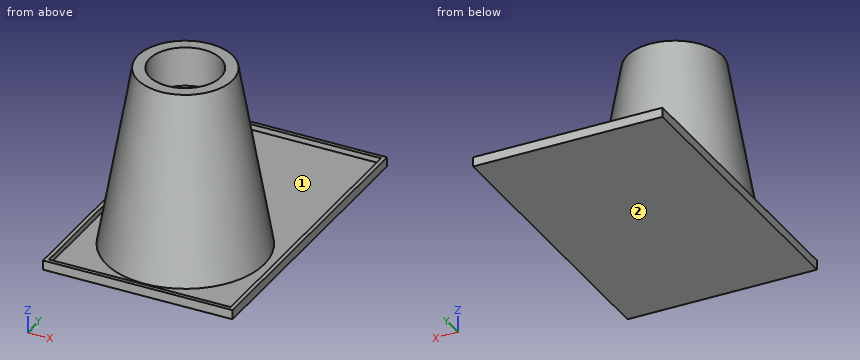
from build123d import *

# Parameters (mm, degrees)
F0_W     = 120
F0_H     = 190
F1_DEPTH = 6
F2_T     = -2.5
F3_R     = 50
F4_DEPTH = 115
F5_SIZE2 = 114.99999
F5_SIZE  = 19.99999
F6_R     = 22.5
F7_DEPTH = 25


# Not quite as in the source:
# - a fillet or chamfer is up to 0.001 mm smaller than in the source, because OpenCascade refuses the exact size


with BuildPart() as f1:
    # F0 (on Top) → F1 (new body)
    with BuildSketch(Plane.XY):
        with Locations((0, 36.5384568274)):
            Rectangle(F0_W, F0_H)
    extrude(amount=F1_DEPTH)

    # F2
    f2_openings = [f1.faces().sort_by_distance(p)[0] for p in [
        (0, 36.538457, 6),
    ]]
    offset(amount=F2_T, openings=f2_openings)

    # F3 (on face) → F4 (join)
    with BuildSketch(Plane.XY.offset(2.5)):
        Circle(F3_R)
    extrude(amount=F4_DEPTH)

    # F5 (size 20 and 115 in the source; OpenCascade refuses exactly that, so slightly less here)
    f5_edges = [f1.edges().sort_by_distance(p)[0] for p in [
        (-50, 0, 117.5),
    ]]
    f5_side = f1.faces().sort_by_distance((0, 0, 117.5))[0]
    chamfer(f5_edges, length=F5_SIZE, length2=F5_SIZE2, reference=f5_side)

    # F6 (on face) → F7 (cut)
    with BuildSketch(Plane.XY.offset(117.5)):
        Circle(F6_R)
    extrude(amount=-F7_DEPTH, mode=Mode.SUBTRACT)


solid = f1.part
The listing builds one solid part. Answer for the finished solid, in the listing's coordinates (mm). Face numbers are marked on the shaded views. Round coordinates to 2 decimals unless told otherwise and drop trailing zeros. Loops run counter-clockwise (first coordinate to the right, second up) from the corner with the lowest first, then second, coordinate; pieces in that order, holes last. Notation, with made-up numbers: M 32.5,65 L 43.5,65 A19 cw 43.5,93 Z; hole C 35.5,33.25 d5. An arc over 180 degrees is marked long. Write each question's results on one line, items separated by ' | '. Start each with the question number.
1) Find section C-C on z = 95. Write down the section's boundary in (x, y).
2) Find section D-D on z = 35. Write down the section's boundary in (x, y).
3) Determine the mould class of the marked faces 1 and 2 for opening direction X: pulls with the +X half, pulls with the -X half, needs draft (parallel to the pull), parting line crosses it, or undercut.
4) Straight lines are drawn through the part: probe 1 along Z at (x, y) = (43, 94.5); probe 2 along Y at (x, z) = (0, 106); probe 3 along Y at (x, z) = (0, 104.75). For each, find the intervals that lie inside material, in ascending order.
5) Each of these flat-tipped pins is pushed along its axis until it touches: pin 1 (5 mm diameter, centred on x = -38, z = 42, fed in from +Y); pin 2 (2 mm diameter, centred on x = 38.5, y = 60.5, fed in from -Z); pin 3 (8 mm diameter, centred on x = 32.5, z = 68, fed in from +Y); pin 4 (1.5 mm diameter, centred on x = 46.5, y = -32.5, fed in from +Z). Where does it stop, or does it pass through?
Final values:
1) outline: C 0,0 d67.83; hole C 0,0 d45
2) outline: C 0,0 d88.7
3) face 1: undercut | face 2: needs draft
4) probe 1: 0 to 2.5 | probe 2: -32 to -22.5, 22.5 to 32 | probe 3: -32.22 to -22.5, 22.5 to 32.22
5) pin 1: y = 24.57 | pin 2: z = 0 | pin 3: y = 26.17 | pin 4: z = 2.5
